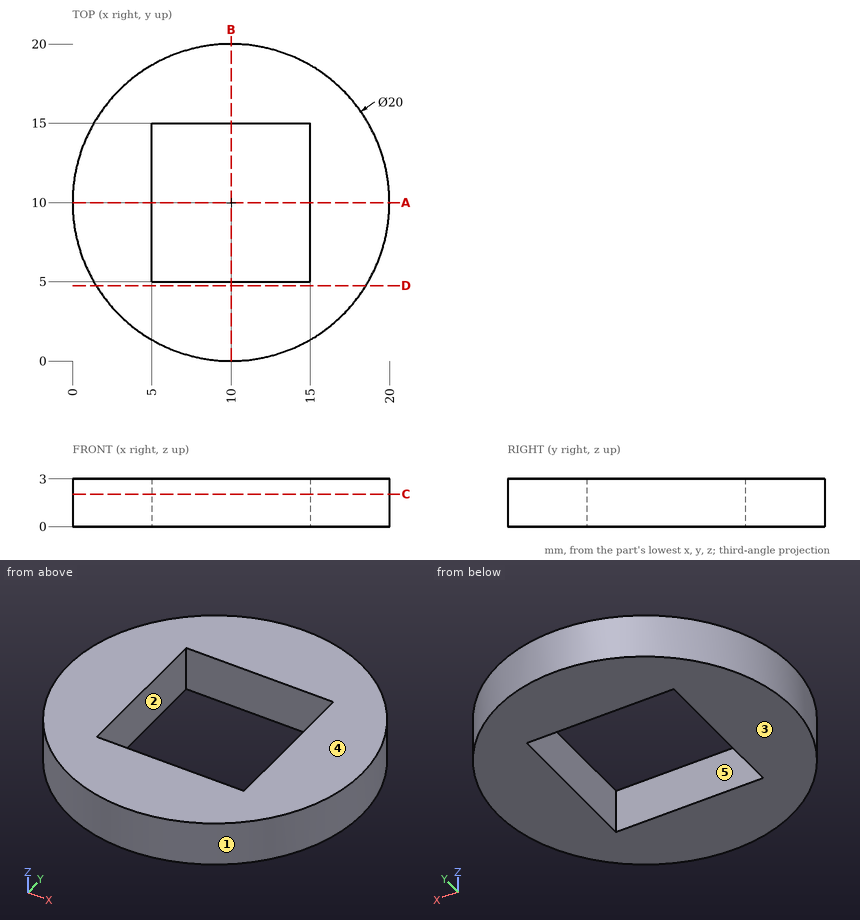
The drawing under review shows one solid part. Ordinate dimensions are in mm from its lowest x, y, z. A direction names the side the tool comes from. Coordinates: 2 decimals unless noted, no trailing zeros. Order: outer loops, then holes, each group sorted by start corner. A loop starts at its lowest first (then second) coordinate and runs counter-clockwise, first axis right, second up. Notation, with made-up numbers: (11.25, -27.5) -> (52.25, -27.5) arc R15 ccw to (52.25, -2.5) -> close; hole circle Ø9 at (17.5, -16.5). An arc over 180 degrees is marked (long way). Answer in a Markdown table with one row per item. Add a question column.
Item 1: To check wall thickness, follow probe 1 along X at (y, z) = (10.5, 2.75); probe 2 along X at (y, z) = (13.5, 2.2). State the ranges of each line that lie inside material, in increasing order.
Item 2: Mouldability with a two-part tool opening along X and no side actions: class the marked faces 1, 2 and 3 as +X half, -X half, draft (parallel to the pull), parting line (faces both ways), or undercut.
Item 3: Machinability: for the marked faces 4 and 5, which of the approach directions +Z, -Z, +X, -X, +Y, -Y give a long, thin tool a straight path to every point of the face, cutting with its end or side? Answer none if there is none.
Item 4: We need section D-D on y = 4.75. Write out the cut boundary in (x, z).
Item 5: We need section C-C on z = 2.05. Write out the cut boundary in (x, y), plus the area to 3 significant figures.
Item 6: Clearance check with a flat-ended pin moving along its axis: pin 1 (1.5 mm diameter, centred on y = 7.5, z = 1, fed in from +X). State where the tip first meets the part, or that it passes through.
Item 7: We need section A-A on y = 10. Write out the cut boundary in (x, z).
Final values:
| question | item | result |
|---|---|---|
| 1 | probe 1 | x = 0.01 to 5, 15 to 19.99 |
| 1 | probe 2 | x = 0.63 to 5, 15 to 19.37 |
| 2 | face 1 | parting line |
| 2 | face 2 | undercut |
| 2 | face 3 | draft |
| 3 | face 4 | +Z, +X, -X, +Y, -Y |
| 3 | face 5 | +Z, -Z |
| 4 | outline | (1.49, 0) -> (18.51, 0) -> (18.51, 3) -> (1.49, 3) -> close |
| 5 | outline | circle Ø20 at (10, 10); hole (5, 5) -> (15, 5) -> (15, 15) -> (5, 15) -> close |
| 5 | area | 214 mm2 |
| 6 | pin 1 | stops at x = 19.85 |
| 7 | outline | (0, 0) -> (5, 0) -> (5, 3) -> (0, 3) -> close; (15, 0) -> (20, 0) -> (20, 3) -> (15, 3) -> close |
